from build123d import *

# Parameters (mm, degrees)
BOSS_EXTRUDE1_DEPTH                               = 3
SKETCH2_W                                         = 36
SKETCH2_H                                         = 30
BOSS_EXTRUDE2_DEPTH                               = 4
CSK_FOR_2_FLAT_HEAD_MACHINE_SCREW_100_D           = 2.4384
CSK_FOR_2_FLAT_HEAD_MACHINE_SCREW_100_CSINK_D     = 4.3688
CSK_FOR_2_FLAT_HEAD_MACHINE_SCREW_100_CSINK_ANGLE = 100


with BuildPart() as part:
    # Sketch1 → Boss-Extrude1 (new body, symmetric)
    with BuildSketch(Plane(origin=(0, 0, 0), x_dir=(0, 0, -1), z_dir=(1, 0, 0))):
        Polygon((4, 26), (9, 26), (9, 16), (13, 16), (13, 30), (0, 30), (0, 0), (4, 0), align=None)
    extrude(amount=BOSS_EXTRUDE1_DEPTH, both=True)

    # Sketch2 → Boss-Extrude2 (add)
    with BuildSketch(Plane.XY):
        with Locations((0, 15)):
            Rectangle(SKETCH2_W, SKETCH2_H)
    extrude(amount=-BOSS_EXTRUDE2_DEPTH)

    # CSK for #2 Flat Head Machine Screw (100)1 (through all)
    with Locations(Plane(origin=(0, 0, -4), x_dir=(-1, 0, 0), z_dir=(0, 0, -1))):
        with Locations((-13, 25), (-13, 5), (13, 5), (13, 25)):
            CounterSinkHole(CSK_FOR_2_FLAT_HEAD_MACHINE_SCREW_100_D / 2, CSK_FOR_2_FLAT_HEAD_MACHINE_SCREW_100_CSINK_D / 2, counter_sink_angle=CSK_FOR_2_FLAT_HEAD_MACHINE_SCREW_100_CSINK_ANGLE)


solid = part.part
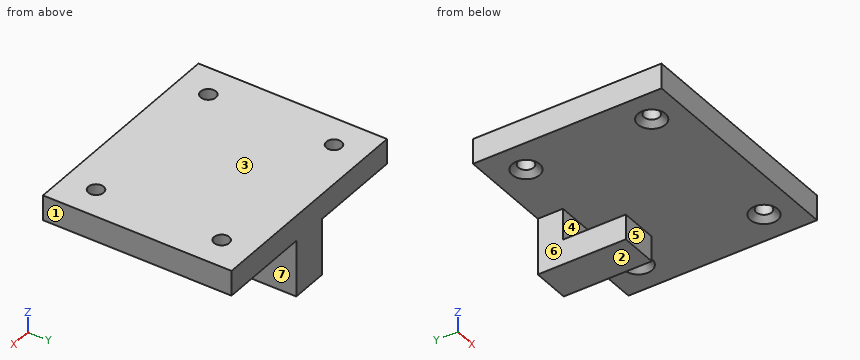
Design review of the part built by this model. Coordinates are the model's own, in mm. Face numbers are marked on the shaded views. A direction names the side the tool comes from. Round coordinates to 2 decimals unless told otherwise and drop trailing zeros. Write each loop counter-clockwise with the first axis right and the second up, starting at its lowest first coordinate (ties: lowest second). Pieces come first, ordered by that corner, then holes.
Item 1: Consider section C-C on z = -2. Give the boundary of the cut face in (x, y).
Item 2: Consider section D-D on y = 19.75. Give the boundary of the cut face in (x, z), and give its area (3 significant figures).
Item 3: Draft analysis for pull direction Z (two halves, no side actions). For the marked faces 1, 2, 3 and 4, state which applies: released by +Z, released by -Z, zero draft, split by the parting line, or undercut.
Item 4: Consider section A-A on x = -13. Give the boundary of the cut face in (y, z), and give its area (3 significant figures).
Item 5: For pin 1 Ø4 at (x, y) = (-13, 5) entering from -Z; pin 2 Ø1.5 at (x, y) = (11, 25) entering from -Z; pin 3 Ø2 at (x, y) = (13, 25) entering from -Z; pin 4 Ø7 at (y, z) = (20, -8) entering from +X, all flat-tipped, find the tip position at first contact; note any pin that passes through.
Item 6: For the marked faces 5, 6 and 7, list the 3-axis set-ups (+Z, -Z, +X, -X, +Y, -Y) from which the entire face can be reached by the end or side of a thin tool; tool diameter is ignored.
Item 7: Wall thickness on L1, parallel to Y at x = -13, z = -1.35; L2, parallel to X at y = 5, z = -1.95; L3, parallel to Z at x = 1, y = 21.25: over which ranges is each line inside the solid? List them lowest first.
Item 8: Consider section B-B on y = 25. Give the boundary of the cut face in (x, z).
Check values:
1. outline: (-18, 0) - (18, 0) - (18, 30) - (-18, 30) - close; hole circle Ø2.44 at (-13, 5); hole circle Ø2.44 at (-13, 25); hole circle Ø2.44 at (13, 5); hole circle Ø2.44 at (13, 25)
2. outline: (-18, -4) - (18, -4) - (18, 0) - (-18, 0) - close; (-3, -13) - (3, -13) - (3, -9) - (-3, -9) - close
2. area: 168 mm2
3. face 1: zero draft
3. face 2: released by -Z
3. face 3: released by +Z
3. face 4: undercut
4. outline: (0, -4) - (2.82, -4) - (3.78, -3.19) - (3.78, 0) - (0, 0) - close; (6.22, -3.19) - (7.18, -4) - (22.82, -4) - (23.78, -3.19) - (23.78, 0) - (6.22, 0) - close; (26.22, -3.19) - (27.18, -4) - (30, -4) - (30, 0) - (26.22, 0) - close
4. area: 98.9 mm2
5. pin 1: stops at z = -3.85
5. pin 2: stops at z = -4
5. pin 3: passes through
5. pin 4: stops at x = 3
6. face 5: -Z, +X, -X, -Y
6. face 6: -Z, -X, +Y, -Y
6. face 7: -Z, +X, +Y, -Y
7. L1: y = 0 to 3.78, 6.22 to 23.78, 26.22 to 30
7. L2: x = -18 to -14.22, -11.78 to 11.78, 14.22 to 18
7. L3: z = -13 to -9, -4 to 0
8. outline: (-18, -4) - (-15.18, -4) - (-14.22, -3.19) - (-14.22, 0) - (-18, 0) - close; (-11.78, -3.19) - (-10.82, -4) - (10.82, -4) - (11.78, -3.19) - (11.78, 0) - (-11.78, 0) - close; (-3, -13) - (3, -13) - (3, -9) - (-3, -9) - close; (14.22, -3.19) - (15.18, -4) - (18, -4) - (18, 0) - (14.22, 0) - close
